```python
from build123d import *
from OCP.BRepFilletAPI import BRepFilletAPI_MakeChamfer

# Parameters (mm, degrees)
BOSS_EXTRUDE1_START     = 1
SKETCH1_R               = 11.9
BOSS_EXTRUDE1_DEPTH     = 10
BOSS_EXTRUDE3_START     = -1
SKETCH1_3_R             = 11.9
BOSS_EXTRUDE3_DEPTH     = 10
SKETCH3_R               = 6
CUT_EXTRUDE1_DEPTH      = 4
SKETCH4_R               = 6
CUT_EXTRUDE2_DEPTH      = 4
BOSS_EXTRUDE9_DEPTH     = 10.5
BOSS_EXTRUDE10_DEPTH    = 3
CHAMFER4_SIZE           = 3
CHAMFER4_SIZE_2         = 5.196152423
CHAMFER5_SIZE           = 3
CHAMFER5_SIZE2          = 6.433520761528718
SKETCH17_R              = 2.500000000000001
SKETCH17_R_2            = 2.500000000000368
SKETCH17_R_3            = 2.5000000000002682
BOSS_EXTRUDE11_DEPTH    = 0.5
BOSS_EXTRUDE12_START    = 0.5
SKETCH18_R              = 2.5000000000000013
SKETCH18_R_2            = 2.5000000000003686
SKETCH18_R_3            = 2.500000000000268
BOSS_EXTRUDE12_DEPTH    = 0.5
CUT_EXTRUDE4_DEPTH      = 59.59880616896635
CHAMFER6_SIZE           = 1.5
SCALE1_SCALE            = 2
SKETCH20_W              = 15
SKETCH20_H              = 6
CUT_EXTRUDE5_DEPTH      = 5
CUT_EXTRUDE8_DEPTH      = 12
CUT_EXTRUDE8_DEPTH_BACK = 8


with BuildPart() as part:
    # Sketch1 → Boss-Extrude1 (new body)
    with BuildSketch(Plane(origin=(0, 0, 0), x_dir=(0, 0, -1), z_dir=(1, 0, 0)).offset(BOSS_EXTRUDE1_START)):
        Circle(SKETCH1_R)
    extrude(amount=BOSS_EXTRUDE1_DEPTH)

    # Sketch4 → Cut-Extrude2 (cut)
    with BuildSketch(Plane.ZY.offset(-1)):
        with Locations(Location((0, 0, 0), (0, 0, 180))):
            Circle(SKETCH4_R)
    extrude(amount=-CUT_EXTRUDE2_DEPTH, mode=Mode.SUBTRACT)



with BuildPart() as body_2:
    # Sketch1<3> → Boss-Extrude3 (new body)
    with BuildSketch(Plane(origin=(0, 0, 0), x_dir=(0, 0, -1), z_dir=(1, 0, 0)).offset(BOSS_EXTRUDE3_START)):
        Circle(SKETCH1_3_R)
    extrude(amount=-BOSS_EXTRUDE3_DEPTH)

    # Sketch3 → Cut-Extrude1 (cut)
    with BuildSketch(Plane(origin=(-1, 0, 0), x_dir=(0, 0, -1), z_dir=(1, 0, 0))):
        Circle(SKETCH3_R)
    extrude(amount=-CUT_EXTRUDE1_DEPTH, mode=Mode.SUBTRACT)


with BuildPart() as part_1:
    add(part.part)

    add(body_2.part)  # Boss-Extrude9 merges body 2
    # Sketch15 → Boss-Extrude9 (add, symmetric)
    with BuildSketch(Plane(origin=(0, 0, 0), x_dir=(0, 0, -1), z_dir=(1, 0, 0))):
        with BuildLine():
            Line((0, 11.9), (19, 11.9))
            Line((19, 11.9), (21.856908233869017, 17.17617999534241))
            Line((21.856908233869017, 17.17617999534241), (27.856908233869014, 17.176179995342412))
            Line((27.856908233869014, 17.176179995342412), (41.084385398468356, 40.17017999534242))
            Line((41.084385398468356, 40.17017999534242), (14.727167600667759, 40.170179995342416))
            Line((14.727167600667759, 40.170179995342416), (-3.657899034187683, 24.74327736286543))
            Line((-3.657899034187683, 24.74327736286543), (-11.182342187352324, 4.070039705575419))
            ThreePointArc((-11.182342187352324, 4.070039705575419), (-6.825559592577466, 9.74790932703899), (0, 11.9))
        make_face()
    extrude(amount=BOSS_EXTRUDE9_DEPTH, both=True)

    # Sketch16 → Boss-Extrude10 (add)
    with BuildSketch(Plane(origin=(0, 4.0700397055754225, 11.182342187352331), x_dir=(1, 0, 0), z_dir=(0, 0.34202014332566566, 0.9396926207859096))):
        Polygon((-10.5, 22.000000000000004), (-10.5, -1.3e-15), (-1, 0), (1, 0), (10.5, -1.3e-15), (10.5, 22.000000000000004), align=None)
    extrude(amount=BOSS_EXTRUDE10_DEPTH)

    # Chamfer4
    chamfer4_edges_1 = [part_1.edges().sort_by_distance(p)[0] for p in [
        (0, 5.096100135552418, 14.00142004971006),
    ]]
    chamfer4_side_1 = [part_1.faces().sort_by_distance(p)[0] for p in [
        (0, 5.075578926952878, 13.945038492462905),
    ]]
    chamfer4_edges_2 = [part_1.edges().sort_by_distance(p)[0] for p in [
        (0, 25.769337792842435, 6.4769768965454135),
    ]]
    chamfer4_side_2 = [part_1.faces().sort_by_distance(p)[0] for p in [
        (0, 25.712956235595282, 6.497498105144953),
    ]]
    chamfer4 = BRepFilletAPI_MakeChamfer(part_1.part.solid().wrapped)
    for e in chamfer4_edges_1:
        chamfer4.Add(CHAMFER4_SIZE - 0.0001, CHAMFER4_SIZE_2 - 0.0001, e.wrapped, chamfer4_side_1[0].wrapped)
    for e in chamfer4_edges_2:
        chamfer4.Add(CHAMFER4_SIZE_2 - 0.0001, CHAMFER4_SIZE - 0.0001, e.wrapped, chamfer4_side_2[0].wrapped)
    add(Compound.cast(chamfer4.Shape()), mode=Mode.REPLACE)  # a hair under: the kernel refuses the full size

    # Chamfer5: one chamfer whose edges measure the first distance from different faces: ONE call of the kernel's chamfer builder (chamfer() names one face for all edges)
    chamfer5_edges_1 = [part_1.edges().sort_by_distance(p)[0] for p in [
        (-10.5, 15.432718964197425, 10.239198473127738),
    ]]
    chamfer5_side_1 = [part_1.faces().sort_by_distance(p)[0] for p in [
        (-10.5, 25.100235238560476, -14.351576366544348),
    ]]
    chamfer5_edges_2 = [part_1.edges().sort_by_distance(p)[0] for p in [
        (10.5, 15.432718964197427, 10.239198473127736),
    ]]
    chamfer5_side_2 = [part_1.faces().sort_by_distance(p)[0] for p in [
        (10.5, 25.100235238560483, -14.35157636654435),
    ]]
    chamfer5 = BRepFilletAPI_MakeChamfer(part_1.part.solid().wrapped)
    for e in chamfer5_edges_1:
        chamfer5.Add(CHAMFER5_SIZE, CHAMFER5_SIZE2, e.wrapped, chamfer5_side_1[0].wrapped)  # the first distance lies on this face
    for e in chamfer5_edges_2:
        chamfer5.Add(CHAMFER5_SIZE, CHAMFER5_SIZE2, e.wrapped, chamfer5_side_2[0].wrapped)  # the first distance lies on this face
    add(Compound.cast(chamfer5.Shape()), mode=Mode.REPLACE)

    # Sketch17 → Boss-Extrude11 (add)
    with BuildSketch(Plane(origin=(11, 0, 0), x_dir=(0, 0, -1), z_dir=(1, 0, 0))):
        with Locations((-4.449357706456068, 5.404)):
            Circle(SKETCH17_R)
        with Locations((6.9046801352792615, 1.1512568043153382)):
            Circle(SKETCH17_R_2)
        with Locations((-2.4553224288227398, -6.5552568043149675)):
            Circle(SKETCH17_R_3)
    extrude(amount=BOSS_EXTRUDE11_DEPTH)

    # Sketch18 → Boss-Extrude12 (add)
    with BuildSketch(Plane.ZY.offset(11).offset(BOSS_EXTRUDE12_START)):
        with Locations(Location((4.449357706456068, 5.404, 0), (0, 0, 180))):
            Circle(SKETCH18_R)
        with Locations(Location((-6.9046801352792615, 1.1512568043153382, 0), (0, 0, 180))):
            Circle(SKETCH18_R_2)
        with Locations(Location((2.4553224288227398, -6.5552568043149675, 0), (0, 0, 180))):
            Circle(SKETCH18_R_3)
    extrude(amount=-BOSS_EXTRUDE12_DEPTH)

    # Sketch19 → Cut-Extrude4 (cut, through all)
    with BuildSketch(Plane.XY):
        Polygon((-4.000000000000002, 40.170179995342416), (4.000000000000002, 40.170179995342416), (4, 29.170179995342412), (-4, 29.170179995342412), align=None)
    extrude(amount=-CUT_EXTRUDE4_DEPTH, mode=Mode.SUBTRACT)

    # Chamfer6
    chamfer6_edges = [part_1.edges().sort_by_distance(p)[0] for p in [
        (-10.5, 40.17017999534242, -27.905776499568056),
        (10.5, 40.17017999534242, -27.905776499568056),
    ]]
    chamfer(chamfer6_edges, length=CHAMFER6_SIZE)


with BuildPart() as part_2:
    # Scale1: scaled about (0, 0, 0)
    add(part_1.part.scale(SCALE1_SCALE))

    # Sketch20 → Cut-Extrude5 (cut)
    with BuildSketch(Plane(origin=(-7.999999999999991, -1.26e-15, 0), x_dir=(0, 0, -1), z_dir=(1, 1.6e-16, 0))):
        with Locations((52.95433520133552, 69.34035999068483)):
            Rectangle(SKETCH20_W, SKETCH20_H)
    cut_extrude5 = extrude(amount=-CUT_EXTRUDE5_DEPTH, mode=Mode.SUBTRACT)

    # Mirror4: Cut-Extrude5 across plane
    add(cut_extrude5.mirror(Plane(origin=(0, 0, 0), x_dir=(0, 0, 1), z_dir=(1, 0, 0))), mode=Mode.SUBTRACT)

    # Sketch21 → Cut-Extrude8 (cut, two sides: drawn at the far end of the back side and taken through both)
    with BuildSketch(Plane(origin=(-2, 0, 0), x_dir=(0, 0, -1), z_dir=(1, 0, 0)).offset(-CUT_EXTRUDE8_DEPTH_BACK)):
        with BuildLine():
            Line((4.835188897605762, -10.982756863578018), (9.589791313584762, -21.78246777942974))
            ThreePointArc((9.589791313584762, -21.78246777942974), (-3.6733884927618106, -23.514808461504543), (-15.776309939282067, -17.819877796991495))
            Line((-15.776309939282067, -17.819877796991495), (-9.625245425797857, -7.166215911703854))
            ThreePointArc((-9.625245425797857, -7.166215911703854), (-3.062295967922119, -11.60268690454276), (4.835188897605762, -10.982756863578018))
        make_face()
    extrude(amount=CUT_EXTRUDE8_DEPTH + CUT_EXTRUDE8_DEPTH_BACK, mode=Mode.SUBTRACT)


solid = part_2.part
```
Could you check a few things on this model? Use its own coordinates, in mm. A direction names the side the tool comes from. Round coordinates to 2 decimals unless told otherwise and drop trailing zeros. Loops run counter-clockwise (first coordinate to the right, second up) from the corner with the lowest first, then second, coordinate; pieces in that order, holes last. Notation, with made-up numbers: M -4.5,41 L 47.5,41 A23 ccw 47.5,64 Z; hole C 51.25,52.5 d4. An arc over 180 degrees is marked long. Write item = value, one per line.
1. Thinking about a two-plate mould opening in Z: for faces 4 (the face through (0.29, 46.54, 10.83)), 5 (the face through (-13, 69, -53)), 6 (the face through (13, 80.34, -56)), which applies, +Z half, -Z half, draft (parallel to the pull), parting line (faces both ways), or undercut?
Results below:
face_4 = +Z half
face_5 = undercut
face_6 = draft
2. I want a section at C-C, the plane z = -67. Write out the boundary of the cut face in (x, y), and give its area (3 significant figures).
Results below:
outline = M -21,53.97 L 21,53.97 L 21,77.34 L 18,80.34 L 8,80.34 L 8,58.34 L -8,58.34 L -8,80.34 L -18,80.34 L -21,77.34 Z
area = 746 mm²
3. Which directions (+Z, -Z, +X, -X, +Y, -Y) give clear straight access to the entire face, cutting with the end or side of a thin tool? Please do faces 1 (the face through (-2, 11.5, -5)), 2 (the face through (-6.056, -12.568, 12.744)), 3 (the face through (5.94, 11.7, -2.66)).
Results below:
face_1 = -Z, -Y
face_2 = -Y
face_3 = none
4. Will these pins go through, and if not, where does the flat tip stop? P1, Ø3.5, axis at x = 9.5, z = -48.5, coming from the -Y side; P2, Ø5, axis at x = 2.5, z = -27, coming from the +Y side; P3, Ø4, axis at x = -12.5, z = -30.5, coming from the -Y side.
Results below:
P1 = 34.35
P2 = 58.34
P3 = 23.8
5. I want a section at D-D, the plane y = 38. Write out the boundary of the cut face in (x, z), and give its area (3 significant figures).
Results below:
outline = M -21,-57.81 L 21,-57.81 L 21,11.5 L 8.13,17.88 L -8.13,17.88 L -21,11.5 Z
area = 3,100 mm²
6. I want a section at A-A, the plane y = -5. Write out the boundary of the cut face in (x, z).
Results below:
outline = M -22,-23.27 L -2,-23.27 L -2,-10.91 L -10,-10.91 L -10,10.91 L -2,10.91 L -2,23.27 L -22,23.27 Z; M 2,-23.27 L 22,-23.27 L 22,23.27 L 2,23.27 L 2,10.91 L 10,10.91 L 10,-10.91 L 2,-10.91 Z
7. I need wall thicknesses on probe 1 along X at (y, z) = (-5.5, -16); probe 2 along Z at (x, y) = (-6.5, 0); probe 3 along X at (y, z) = (65, -54.5). Which ranges of each line are inside material? Lowest first, please.
Results below:
probe_1 = -22 to -2, 2 to 22
probe_2 = -23.8 to -12, 12 to 23.8
probe_3 = -21 to -8, 8 to 21
